Source: CAD feature listing. Evaluate the final solid. Frame: model axes, mm. A direction names the side the tool comes from. Give positions to 0.01 mm unless a question says otherwise; leave off trailing zeros. Write each loop counter-clockwise with the first axis right and the second up, starting at its lowest first coordinate (ties: lowest second). Pieces come first, ordered by that corner, then holes. Notation, with made-up numbers: (44, 12) -> (103, 12) arc R25 cw to (103, 36) -> close; hole circle Ø10 at (75.5, 3). An arc over 180 degrees is marked (long way). Answer as a JSON object with one key per item and string values. Group by question number.
Item 1: Ray query, probe 1 along Y at (x, z) = (0, 1.4); probe 2 along Z at (x, y) = (-8, -2.75); probe 3 along Y at (x, z) = (6.25, 1.95). Return the intervals inside material, ascending. Write a range as from..to.
Item 2: Access query for faces 4 (the face through (1.2, -1.2, 1.5)), 5 (the face through (-5.5, 0.07, 0.99)). Directions: +Z, -Z, +X, -X, +Y, -Y. A direction counts if a zero-diameter tool reaches every point of the face in a straight line with its end or side. Return the directions, or none.
Item 3: Section query A-A on y = 7. Return the cut outline in (x, z).
Item 4: Section query C-C on x = 0. Return the cut outline in (y, z).
Item 5: Pull-direction query (Y, two-part tool) for faces 1 (the face through (-2.17, -9.76, 0.99)), 2 (the face through (0, -2, 0)), 3 (the face through (0.325, -8.464, 0.986)); classes: pulls with the +Y half, pulls with the -Y half, needs draft (parallel to the pull), parting line crosses it, or undercut.
Item 6: First-contact query: pin 1 Ø1.5 at (x, y) = (7.5, -0.5) entering from +Z; pin 2 Ø3.5 at (x, y) = (7, 0) entering from +Z. Flat tips, straight axial feed; report the tip coordinate or a pass-through.
Item 7: Section query D-D on z = 2.55. Return the cut outline in (x, y).
from build123d import *

# Parameters (mm, degrees)
SKETCH_1_R          = 10
EXTRUDE_1_DEPTH     = 2
SKETCH_3_R          = 4.5
EXTRUDE_2_DEPTH     = 2.5
SKETCH_4_R          = 1.5
CUT_EXTRUDE_1_DEPTH = 15.84082208
SKETCH_5_R          = 2.75
CUT_EXTRUDE_2_DEPTH = 3
CHAMFER_1_SIZE      = 0.5
SKETCH_6_R          = 1.5
CUT_EXTRUDE_3_DEPTH = 15.84082208


with BuildPart() as part:
    # 草图1 → 凸台-拉伸1 (new body)
    with BuildSketch(Plane.XY):
        Circle(SKETCH_1_R)
    extrude(amount=EXTRUDE_1_DEPTH)

    # 草图3 → 凸台-拉伸2 (add)
    with BuildSketch(Plane.XY.offset(2)):
        Circle(SKETCH_3_R)
    extrude(amount=EXTRUDE_2_DEPTH)

    # 草图4 → 切除-拉伸1 (cut, through all)
    with BuildSketch(Plane.XY.offset(4.5)):
        Circle(SKETCH_4_R)
    extrude(amount=-CUT_EXTRUDE_1_DEPTH, mode=Mode.SUBTRACT)

    # 草图5 → 切除-拉伸2 (cut)
    with BuildSketch(Plane.XY.offset(4.5)):
        Circle(SKETCH_5_R)
    extrude(amount=-CUT_EXTRUDE_2_DEPTH, mode=Mode.SUBTRACT)

    # 倒角1
    chamfer_1_edges = [part.edges().sort_by_distance(p)[0] for p in [
        (-2.75, 0, 4.5),
    ]]
    chamfer(chamfer_1_edges, length=CHAMFER_1_SIZE)

    # 草图6 → 切除-拉伸3 (cut, through all)
    with BuildSketch(Plane(origin=(0, 0, 0), x_dir=(-1, 0, 0), z_dir=(0, 0, -1))):
        with Locations((-7, 0)):
            Circle(SKETCH_6_R)
        with Locations((0, 7)):
            Circle(SKETCH_6_R)
        with Locations((7, 0)):
            Circle(SKETCH_6_R)
        with Locations((0, -7)):
            Circle(SKETCH_6_R)
    extrude(amount=-CUT_EXTRUDE_3_DEPTH, mode=Mode.SUBTRACT)


solid = part.part
Worked answers:
{
 "1": {"probe 1": "-10..-8.5, -5.5..-1.5, 1.5..5.5, 8.5..10", "probe 2": "0..2", "probe 3": "-7.81..-1.3, 1.3..7.81"},
 "2": {"face 4": "+Z", "face 5": "+Z, -Z"},
 "3": {"outline": "(-7.14, 0) -> (-1.5, 0) -> (-1.5, 2) -> (-7.14, 2) -> close; (1.5, 0) -> (7.14, 0) -> (7.14, 2) -> (1.5, 2) -> close"},
 "4": {"outline": "(-10, 0) -> (-8.5, 0) -> (-8.5, 2) -> (-10, 2) -> close; (-5.5, 0) -> (-1.5, 0) -> (-1.5, 1.5) -> (-2.75, 1.5) -> (-2.75, 4) -> (-3.25, 4.5) -> (-4.5, 4.5) -> (-4.5, 2) -> (-5.5, 2) -> close; (1.5, 0) -> (5.5, 0) -> (5.5, 2) -> (4.5, 2) -> (4.5, 4.5) -> (3.25, 4.5) -> (2.75, 4) -> (2.75, 1.5) -> (1.5, 1.5) -> close; (8.5, 0) -> (10, 0) -> (10, 2) -> (8.5, 2) -> close"},
 "5": {"face 1": "parting line crosses it", "face 2": "needs draft", "face 3": "undercut"},
 "6": {"pin 1": "through", "pin 2": "z = 2"},
 "7": {"outline": "circle Ø9 at (0, 0); hole circle Ø5.5 at (0, 0)"}
}
